Check sheet for the drawn part. Datum: minimum x, y, z corner. Units: mm. Coordinates: 2 decimals unless noted, no trailing zeros. Write each loop counter-clockwise with the first axis right and the second up, starting at its lowest first coordinate (ties: lowest second). Pieces come first, ordered by that corner, then holes. Notation, with made-up numbers: (58.25, -29) -> (67.25, -29) arc R25 cw to (67.25, 9) -> close; hole circle Ø7 at (74.5, 77). An arc over 180 degrees is marked (long way). Answer in a Markdown table with one row per item. Add a question column.
1. Cross-section at C-C on z = 7. Record the cut outline in (x, y), and give its area (3 significant figures).
2. Depth check by flat-ended pin: P1, Ø1.5, axis at x = 11.5, y = 1.5, coming from the -Z side; P2, Ø1, axis at x = 47, y = 2, coming from the -Z side; P3, Ø1.5, axis at x = 62.5, y = 3.5, coming from the -Z side; P4, Ø1.5, axis at y = 2, z = 80, coming from the -X side. Enter the tip coordinate at first touch or a pass-through.
3. Cross-section at A-A on x = 25. Record the cut outline in (y, z), and give its area (3 significant figures).
4. Cross-section at D-D on x = 48.5. Record the cut outline in (y, z), and give its area (3 significant figures).
5. Scan lines: L1, parallel to Z at x = 6.5, y = 1.8; L2, parallel to X at y = 3.45, z = 49; L3, parallel to X at y = 2.7, z = 43.5. Record each from-to range of solid material in increasing order. Write a range as from..to.
6. Cross-section at B-B on y = 2.75. Record the cut outline in (x, z).
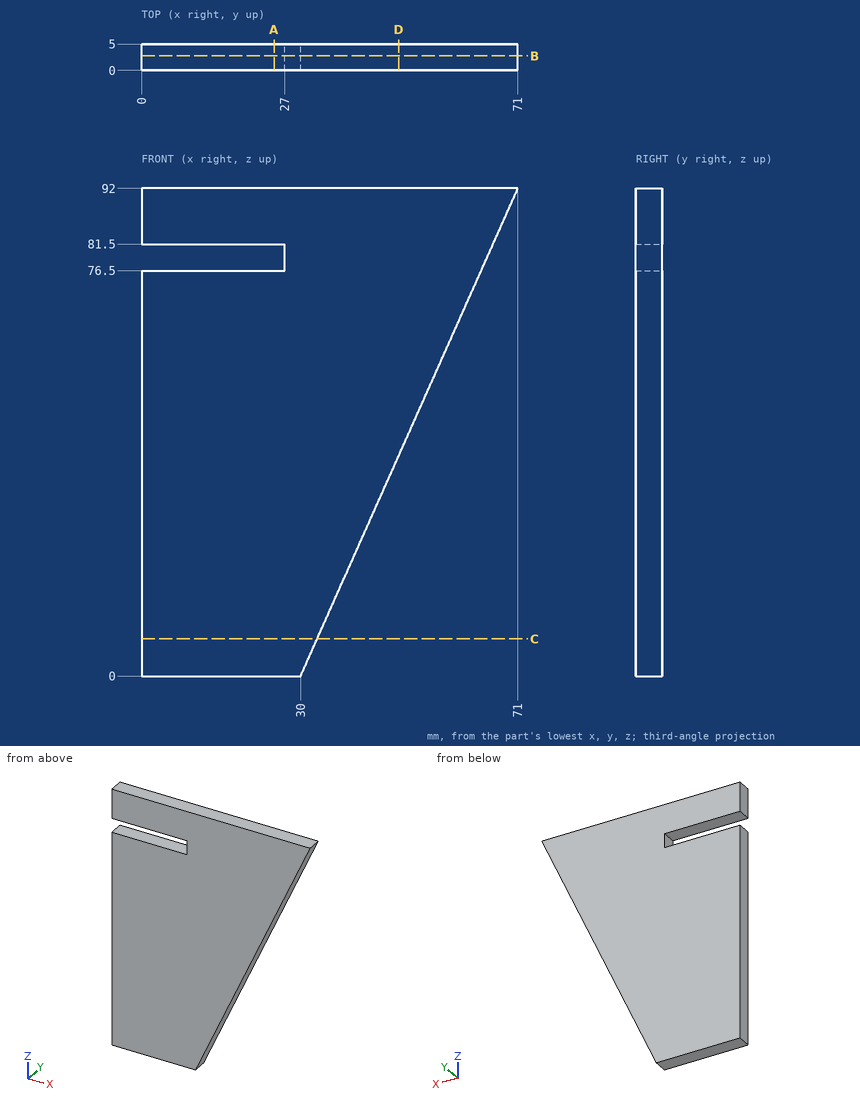
Results found:
| question | item | result |
|---|---|---|
| 1 | outline | (0, 0) -> (33.12, 0) -> (33.12, 5) -> (0, 5) -> close |
| 1 | area | 166 mm^2 |
| 2 | P1 | stops at z = 0 |
| 2 | P2 | stops at z = 37.02 |
| 2 | P3 | stops at z = 71.24 |
| 2 | P4 | stops at x = 27 |
| 3 | outline | (0, 0) -> (5, 0) -> (5, 76.5) -> (0, 76.5) -> close; (0, 81.5) -> (5, 81.5) -> (5, 92) -> (0, 92) -> close |
| 3 | area | 435 mm^2 |
| 4 | outline | (0, 41.51) -> (5, 41.51) -> (5, 92) -> (0, 92) -> close |
| 4 | area | 252 mm^2 |
| 5 | L1 | z = 0..76.5, 81.5..92 |
| 5 | L2 | x = 0..51.84 |
| 5 | L3 | x = 0..49.39 |
| 6 | outline | (0, 0) -> (30, 0) -> (71, 92) -> (0, 92) -> (0, 81.5) -> (27, 81.5) -> (27, 76.5) -> (0, 76.5) -> close |
